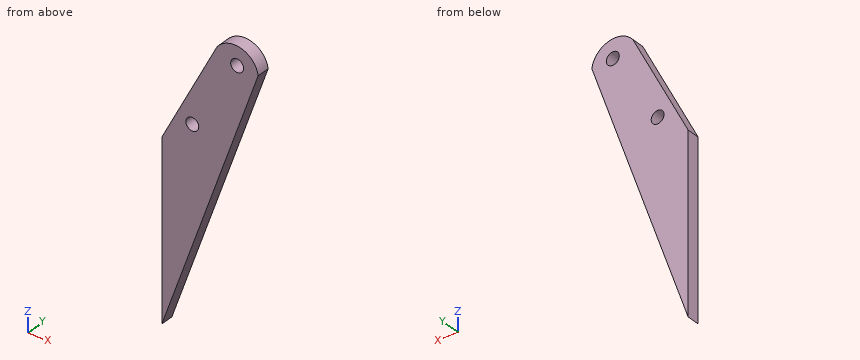
```python
from build123d import *

# Parameters (mm, degrees)
SKETCH1_R           = 1.5
BOSS_EXTRUDE1_DEPTH = 3


with BuildPart() as part:
    # Sketch1 → Boss-Extrude1 (new body)
    with BuildSketch(Plane(origin=(0, 0, 0), x_dir=(1, 0, 0), z_dir=(0, 1, 0))):
        with BuildLine():
            Line((-22.443608406, 63.945737479), (-22.443608406, 22.705737479))
            Line((-22.443608406, 22.705737479), (-9.573677497, -2.498525621))
            ThreePointArc((-9.573677497, -2.498525621), (-3.954490329, -4.438597859), (0, 0))
            Line((0, 0), (-22.443608406, 63.945737479))
        make_face()
        with Locations(Location((-15.336480405, 16.958709415, 0), (0, 0, 270))):
            Circle(SKETCH1_R, mode=Mode.SUBTRACT)
        with Locations(Location((-4.897949582, -0.229925617, 0), (0, 0, 270))):
            Circle(SKETCH1_R, mode=Mode.SUBTRACT)
    extrude(amount=BOSS_EXTRUDE1_DEPTH)


solid = part.part
```
Can you work these out from the model? Positions are in its coordinate system, mm. Give positions to 0.01 mm unless a question says otherwise; leave off trailing zeros. Loops run counter-clockwise (first coordinate to the right, second up) from the corner with the lowest first, then second, coordinate; pieces in that order, holes last. Notation, with made-up numbers: M 33.5,16.25 L 78.5,16.25 A11 cw 78.5,30.25 Z; hole C 56.5,15.25 d6. An arc over 180 degrees is marked long. Answer in a Markdown table with one row per item.
1. If I drill on line 1 along X through (y, z) = (1.55, -9); line 2 along X through (y, z) = (2.6, -40), over which ranges is the centre line in solid material (lowest first)?
Taken from the geometry:
| item | result |
|---|---|
| line 1 | x = -15.45 to -3.16 |
| line 2 | x = -22.44 to -14.04 |
2. Suppose I cut it at A-A on x = -4. Write out the boundary of the cut face in (y, z).
Taken from the geometry:
| item | result |
|---|---|
| outline | M 0,-11.4 L 3,-11.4 L 3,-0.97 L 0,-0.97 Z; M 0,1.43 L 3,1.43 L 3,4.45 L 0,4.45 Z |
3. Suppose I cut it at B-B on y = 0.45. Write out the boundary of the cut face in (x, z), plus the area to 3 significant figures.
Taken from the geometry:
| item | result |
|---|---|
| outline | M -22.44,-63.95 L 0,0 A5.36 ccw -9.57,2.5 L -22.44,-22.71 Z; hole C -15.34,-16.96 d3; hole C -4.9,0.23 d3 |
| area | 609 mm² |
4. Suppose I cut it at D-D on z = -5. Write out the boundary of the cut face in (x, y), plus the area to 3 significant figures.
Taken from the geometry:
| item | result |
|---|---|
| outline | M -13.4,0 L -1.75,0 L -1.75,3 L -13.4,3 Z |
| area | 34.9 mm² |
5. Suppose I cut it at C-C on x = -14.5. Write out the boundary of the cut face in (y, z).
Taken from the geometry:
| item | result |
|---|---|
| outline | M 0,-41.31 L 3,-41.31 L 3,-18.2 L 0,-18.2 Z; M 0,-15.71 L 3,-15.71 L 3,-7.15 L 0,-7.15 Z |
6. For pin 1 Ø4 at (x, z) = (-15.34, -16.96) entering from +Y; pin 2 Ø2.5 at (x, z) = (-4.9, 0.23) entering from +Y, each with a flat end and sliding along its axis, tell me the tip position at first contact or that it passes through.
Taken from the geometry:
| item | result |
|---|---|
| pin 1 | stops at y = 3 |
| pin 2 | passes through |
